The listing builds one solid part. Answer for the finished solid, in the listing's coordinates (mm). A direction names the side the tool comes from. Coordinates: 2 decimals unless noted, no trailing zeros. Order: outer loops, then holes, each group sorted by start corner. A loop starts at its lowest first (then second) coordinate and runs counter-clockwise, first axis right, second up. Notation, with made-up numbers: (54, -15) -> (78, -15) arc R22 ccw to (78, 18) -> close; hole circle Ø8 at (-6, -3.5). An arc over 180 degrees is marked (long way). Return JSON: item names as keys, results as strings.
from build123d import *

# Parameters (mm, degrees)
F0_W     = 27.65
F0_H     = 15
F1_DEPTH = 15
F3_DEPTH = 7.366
F4_DEPTH = 40
F6_DEPTH = 7.366
F7_R     = 12
F8_R     = 2
F9_DEPTH = 30


with BuildPart() as f1:
    # F0 (on Front) → F1 (new body, symmetric)
    with BuildSketch(Plane.XZ):
        Polygon((-6.175, -27.5), (13.825, -27.5), (13.825, 27.5), (-13.825, 27.5), (-13.825, -5.5), (-13.825, -27.5), (-9.825, -27.5), (-9.825, -5.5), (-6.175, -5.5), align=None)
        with Locations((0, 35)):
            Rectangle(F0_W, F0_H)
    extrude(amount=F1_DEPTH, both=True)

    # F2 (on face) → F3 (cut)
    with BuildSketch(Plane.YZ.offset(13.825)):
        with BuildLine():
            ThreePointArc((11.1125, 27.5), (7.8577241059, 35.3577241059), (0, 38.6125))
            ThreePointArc((0, 38.6125), (-7.8577241059, 19.6422758941), (11.1125, 27.5))
        make_face()
        with BuildLine():
            ThreePointArc((8.89, 27.5), (-6.2861792847, 21.2138207153), (0, 36.39))
            ThreePointArc((0, 36.39), (6.2861792847, 33.7861792847), (8.89, 27.5))
        make_face(mode=Mode.SUBTRACT)
    extrude(amount=-F3_DEPTH, mode=Mode.SUBTRACT)

    # F4 (cut): a face of the model
    f4_faces = [f1.faces().sort_by_distance(p)[0] for p in [
        (13.825, 0, 27.5),
    ]]
    extrude(f4_faces, amount=-F4_DEPTH, mode=Mode.SUBTRACT)

    # F5 (on face) → F6 (cut)
    with BuildSketch(Plane(origin=(-13.825, 0, 0), x_dir=(0, -1, 0), z_dir=(-1, 0, 0))):
        with BuildLine():
            ThreePointArc((11.2, 27.5), (7.9195959493, 35.4195959493), (0, 38.7))
            ThreePointArc((0, 38.7), (-7.9195959493, 19.5804040507), (11.2, 27.5))
        make_face()
        with BuildLine():
            ThreePointArc((8.89, 27.5), (-6.2861792847, 21.2138207153), (0, 36.39))
            ThreePointArc((0, 36.39), (6.2861792847, 33.7861792847), (8.89, 27.5))
        make_face(mode=Mode.SUBTRACT)
    extrude(amount=-F6_DEPTH, mode=Mode.SUBTRACT)

    # F7
    f7_edges = [f1.edges().sort_by_distance(p)[0] for p in [
        (0, 15, 42.5),
        (0, -15, 42.5),
    ]]
    fillet(f7_edges, radius=F7_R)

    # F8 (on face) → F9 (cut)
    with BuildSketch(Plane(origin=(-13.825, 0, 0), x_dir=(0, -1, 0), z_dir=(-1, 0, 0))):
        with BuildLine():
            Line((-2, -16.5), (0, -16.5))
            Line((0, -16.5), (2, -16.5))
            ThreePointArc((2, -16.5), (0, -14.5), (-2, -16.5))
        make_face()
        with BuildLine():
            ThreePointArc((-2, -16.5), (-1.4142135624, -17.9142135624), (0, -18.5))
            Line((0, -18.5), (0, -16.5))
            Line((0, -16.5), (-2, -16.5))
        make_face()
        with BuildLine():
            Line((0, -16.5), (0, -18.5))
            ThreePointArc((0, -18.5), (1.4142135624, -17.9142135624), (2, -16.5))
            Line((2, -16.5), (0, -16.5))
        make_face()
        with Locations((-8, -16.5)):
            Circle(F8_R)
        with BuildLine():
            ThreePointArc((10, -16.5), (8, -14.5), (6, -16.5))
            ThreePointArc((6, -16.5), (8, -18.5), (10, -16.5))
        make_face()
    extrude(amount=-F9_DEPTH, mode=Mode.SUBTRACT)


solid = f1.part
1. Each of these flat-tipped pins is pushed along its axis until it touches: pin 1 Ø1.8 at (x, y) = (-7.5, -1) entering from -Z; pin 2 Ø10.5 at (y, z) = (0, 27.5) entering from -X; pin 3 Ø6 at (x, y) = (-8, -9) entering from +Z; pin 4 Ø18 at (y, z) = (0.5, 25.5) entering from +X. Where does it stop, or does it pass through?
Answer block:
{"pin 1": "stops at z = -5.5", "pin 2": "passes through", "pin 3": "stops at z = 42.12", "pin 4": "stops at x = 6.46"}
2. Consider line 1 (Y direction, x = 8.5, z = 27); line 2 (X direction, y = 3.5, z = -23.5) (3 decimals); line 3 (Z direction, x = -8, y = 0.5). Determine where each line is inside the solid, lowest interval first. Write a range as from..to.
Answer block:
{"line 1": "y = -15..-11.1, 11.1..15", "line 2": "x = -13.825..-9.825, -6.175..13.825", "line 3": "z = -5.5..16.31, 38.69..42.5"}
3. The part is cut by section A-A on x = -1.75. Give the vertices of the cut face in (y, z), and give its area (3 significant figures).
Answer block:
{"outline": "(-15, -27.5) -> (15, -27.5) -> (15, 30.5) arc R12 ccw to (3, 42.5) -> (-3, 42.5) arc R12 ccw to (-15, 30.5) -> close; hole circle Ø4 at (-8, -16.5); hole circle Ø17.78 at (0, 27.5); hole circle Ø4 at (0, -16.5); hole circle Ø4 at (8, -16.5)", "area": "1,750 mm2"}
4. The part is cut by section D-D on y = -7. Give the vertices of the cut face in (x, z) (3 decimals).
Answer block:
{"outline": "(-13.825, -27.5) -> (-9.825, -27.5) -> (-9.825, -18.232) -> (-13.825, -18.232) -> close; (-13.825, -14.768) -> (-9.825, -14.768) -> (-9.825, -5.5) -> (-6.175, -5.5) -> (-6.175, -14.768) -> (13.825, -14.768) -> (13.825, 18.869) -> (6.459, 18.869) -> (6.459, 22.02) -> (-6.459, 22.02) -> (-6.459, 18.757) -> (-13.825, 18.757) -> close; (-13.825, 36.243) -> (-6.459, 36.243) -> (-6.459, 32.98) -> (6.459, 32.98) -> (6.459, 36.131) -> (13.825, 36.131) -> (13.825, 41.814) -> (-13.825, 41.814) -> close; (-6.175, -27.5) -> (13.825, -27.5) -> (13.825, -18.232) -> (-6.175, -18.232) -> close"}
5. For faces 4 (the face through (-6.459, 8, 33)), 5 (the face through (-9.825, 0, -14)), 6 (the face through (6.459, 0, 37)), 7 (the face through (0.19, -11.58, 38.89)), 8 (the face through (3.685, 8.26, -14.517)), determine the directions among +Z, -Z, +X, -X, +Y, -Y from which every point of the face is accessible in a straight line to the end or side of a thin tool.
Answer block:
{"face 4": "-X", "face 5": "-Z, +Y, -Y", "face 6": "+X", "face 7": "+Z, +X, -X, -Y", "face 8": "+X, -X"}
6. The part is cut by section B-B on x = -7.75. Give the vertices of the cut face in (y, z).
Answer block:
{"outline": "(-15, -5.5) -> (15, -5.5) -> (15, 30.5) arc R12 ccw to (3, 42.5) -> (-3, 42.5) arc R12 ccw to (-15, 30.5) -> close; hole circle Ø22.4 at (0, 27.5)"}
7. Determine the mould class of faces 1 (the face through (-11.853, 8.26, -14.517)), 2 (the face through (0, -15, 2)), 3 (the face through (0, 15, 2)) for opening direction Y: pulls with the +Y half, pulls with the -Y half, needs draft (parallel to the pull), parting line crosses it, or undercut.
Answer block:
{"face 1": "undercut", "face 2": "pulls with the -Y half", "face 3": "pulls with the +Y half"}
8. The part is cut by section C-C on y = 1. Give the vertices of the cut face in (x, z) (3 decimals).
Answer block:
{"outline": "(-13.825, -27.5) -> (-9.825, -27.5) -> (-9.825, -18.232) -> (-13.825, -18.232) -> close; (-13.825, -14.768) -> (-9.825, -14.768) -> (-9.825, -5.5) -> (-6.175, -5.5) -> (-6.175, -14.768) -> (13.825, -14.768) -> (13.825, 16.433) -> (6.459, 16.433) -> (6.459, 18.666) -> (-6.459, 18.666) -> (-6.459, 16.345) -> (-13.825, 16.345) -> close; (-13.825, 38.655) -> (-6.459, 38.655) -> (-6.459, 36.334) -> (6.459, 36.334) -> (6.459, 38.567) -> (13.825, 38.567) -> (13.825, 42.5) -> (-13.825, 42.5) -> close; (-6.175, -27.5) -> (13.825, -27.5) -> (13.825, -18.232) -> (-6.175, -18.232) -> close"}
